```python
from build123d import *

# Parameters (mm, degrees)
SKETCH1_W           = 27.3
SKETCH1_H           = 12.3
BOSS_EXTRUDE1_DEPTH = 23.5
SKETCH3_W           = 30.4
SKETCH3_H           = 14
BOSS_EXTRUDE2_DEPTH = 2
SKETCH4_W           = 22.788352984
SKETCH4_H           = 8.421389372
BOSS_EXTRUDE3_DEPTH = 5
CUT_EXTRUDE2_START  = -8.421389371
CUT_EXTRUDE2_DEPTH  = 8.421389371


# Read off the part's stored shape, not the designer's step: Cut-Extrude2
with BuildPart() as part:
    # Sketch1 → Boss-Extrude1 (new body)
    with BuildSketch(Plane(origin=(0, 0, 0), x_dir=(1, 0, 0), z_dir=(0, 1, 0))):
        Rectangle(SKETCH1_W, SKETCH1_H)
    extrude(amount=BOSS_EXTRUDE1_DEPTH)

    # Sketch3 → Boss-Extrude2 (add)
    with BuildSketch(Plane(origin=(0, 23.5, 0), x_dir=(1, 0, 0), z_dir=(0, 1, 0))):
        Rectangle(SKETCH3_W, SKETCH3_H)
    extrude(amount=BOSS_EXTRUDE2_DEPTH)

    # Sketch4 → Boss-Extrude3 (add)
    with BuildSketch(Plane(origin=(0, 25.5, 0), x_dir=(1, 0, 0), z_dir=(0, 1, 0))):
        Rectangle(SKETCH4_W, SKETCH4_H)
    extrude(amount=BOSS_EXTRUDE3_DEPTH)

    # Cut-Extrude2 outline → Cut-Extrude2 (cut)
    with BuildSketch(Plane.XY.offset(4.210694686).offset(CUT_EXTRUDE2_START)):
        with BuildLine():
            ThreePointArc((-11.394176492, 25.5), (-10.180313992, 28.04843269), (-8.781103834, 30.5))
            Line((-8.781103834, 30.5), (-11.394176492, 30.5))
            Line((-11.394176492, 30.5), (-11.394176492, 25.5))
        make_face()
        with BuildLine():
            ThreePointArc((-8.781103834, 30.5), (1.034220457, 27.1323045), (11.394176492, 26.537935189))
            Line((11.394176492, 26.537935189), (11.394176492, 30.5))
            Line((11.394176492, 30.5), (-8.781103834, 30.5))
        make_face()
    extrude(amount=CUT_EXTRUDE2_DEPTH, mode=Mode.SUBTRACT)


solid = part.part
```
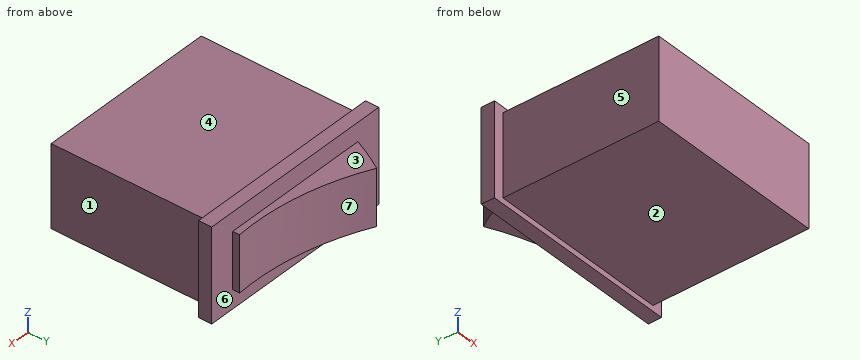
Model file for the job. Use its own axes, mm. Face numbers are marked on the shaded views. A direction names the side the tool comes from. Give positions to 0.01 mm unless a question says otherwise; leave off trailing zeros. Loops run counter-clockwise (first coordinate to the right, second up) from the corner with the lowest first, then second, coordinate; pieces in that order, holes last. Notation, with made-up numbers: M 16.5,84.25 L 42.5,84.25 A14 ccw 42.5,101.25 Z; hole C -9.5,21 d6. An arc over 180 degrees is marked long. Use one line per item in the form item = value.
Item 1: Slice it at C-C on z = 5. List the corners of the cut face in (x, y), and give its area (3 significant figures).
Filled in:
outline = M -15.2,23.5 L -13.65,23.5 L -13.65,0 L 13.65,0 L 13.65,23.5 L 15.2,23.5 L 15.2,25.5 L -15.2,25.5 Z
area = 702 mm^2
Item 2: Slice it at B-B on x = 8. List the corners of the cut face in (y, z).
Filled in:
outline = M 0,-6.15 L 23.5,-6.15 L 23.5,-7 L 25.5,-7 L 25.5,-4.21 L 26.42,-4.21 L 26.42,4.21 L 25.5,4.21 L 25.5,7 L 23.5,7 L 23.5,6.15 L 0,6.15 Z
Item 3: Slice it at A-A on z = 2.5. List the corners of the cut face in (x, y).
Filled in:
outline = M -15.2,23.5 L -13.65,23.5 L -13.65,0 L 13.65,0 L 13.65,23.5 L 15.2,23.5 L 15.2,25.5 L 11.39,25.5 L 11.39,26.54 A38.1 cw -8.78,30.5 A38.1 ccw -11.39,25.5 L -15.2,25.5 Z
Item 4: Flat gauge pins, fed straight in: pin 1 Ø2 at (x, y) = (1.5, 5.5) entering from -Z; pin 2 Ø0.8 at (y, z) = (26, 1) entering from +X; pin 3 Ø8 at (x, z) = (-3, -3) entering from +Y. Where does each tip first touch, or does it go through?
Filled in:
pin_1 = -6.15
pin_2 = 11.39
pin_3 = 29.66
Item 5: Two-plate mould, pull along X, no slides. Class the marked faces 5, 6 and 7: released by +X, released by -X, zero draft, split by the parting line, or undercut.
Filled in:
face_5 = released by -X
face_6 = zero draft
face_7 = undercut
Item 6: Which spindle directions (+Z, -Z, +X, -X, +Y, -Y) get a long thin tool onto all of the face, cutting with end or side? Do the marked faces 1, 2, 3 and 4. Say none if no direction does.
Filled in:
face_1 = +Z, -Z, +X, -Y
face_2 = -Z, +X, -X, -Y
face_3 = +Z, +X, -X, +Y
face_4 = +Z, +X, -X, -Y
Item 7: Slice it at D-D on y = 6.5. List the corners of the cut face in (x, z).
Filled in:
outline = M -13.65,-6.15 L 13.65,-6.15 L 13.65,6.15 L -13.65,6.15 Z
Item 8: Drill centre lines: L1, parallel to X at y = 12, z = 2.5; L2, parallel to Z at x = -11.5, y = 14.5; L3, parallel to Y at x = -13.5, z = -3.25. Where is each one in solid material? Low to high.
Filled in:
L1 = -13.65 to 13.65
L2 = -6.15 to 6.15
L3 = 0 to 25.5
